Read the model definition and answer for the solid it produces. Units are mm, in the model's axes. A direction names the side the tool comes from. Give positions to 0.01 mm unless a question says otherwise; leave off trailing zeros. Write each loop counter-clockwise with the first axis right and the second up, starting at its lowest first coordinate (ties: lowest second). Pieces come first, ordered by that corner, then holes. Notation, with made-up numbers: (40, 23.5) -> (67, 23.5) arc R17 cw to (67, 37.5) -> close; hole circle Ø2 at (-40, 40.5). An arc over 180 degrees is marked (long way). Answer as CSV lines item,"result". Start each with the question number.
1. Given pin 1 (1.5 mm diameter, centred on x = 151.5, y = 38.5, fed in from -Z), flat-ended and moving along its own axis, determine where the tip first touches the part or whether it passes through.
2. The part is cut by section B-B, the plane y = 27.5. Determine the outline of the cut face in (x, z).
3. A tool of negligible diameter and unlimited length cuts with its end or side. For faces 4 (the flat face through (76, 77, 4)), 5 (the flat face through (92, 72, 3)), 6 (the cylindrical face through (40.455, 74.535, 4.354)), from which of +Z, -Z, +X, -X, +Y, -Y can it reach the whole face along a straight path? Write none if from no direction.
4. The part is cut by section A-A, the plane x = 121.5. Determine the outline of the cut face in (y, z), and give its area (3 significant figures).
5. For a pull along Y with two mould halves and no side action, classify faces 1 (the flat face through (0, 38, 4)), 2 (the flat face through (78.25, 39, 3)), 3 (the flat face through (76, 0, 4)) as pulls with the +Y half, pulls with the -Y half, needs draft (parallel to the pull), parting line crosses it, or undercut.
6. Find the intervals of material crossed by line 1 (X direction, y = 51, z = 4.5); line 2 (Y direction, x = 126.25, z = 3.2); line 3 (Y direction, x = 151.5, z = 3.85), in increasing order.
from build123d import *

# Parameters (mm, degrees)
F0_W      = 154
F0_H      = 77
F1_DEPTH  = 8.127
F3_R      = 1.25
F4_DEPTH  = 5
F5_R      = 1.25
F6_DEPTH  = 5
F7_R      = 1.25
F8_DEPTH  = 5
F9_R      = 1.25
F10_DEPTH = 5
F11_R     = 1.25
F12_DEPTH = 5
F13_R     = 1.25
F14_DEPTH = 5
F15_R     = 1.25
F16_DEPTH = 5
F17_R     = 1.25
F18_DEPTH = 5
F19_R     = 1.25
F20_DEPTH = 5
F21_R     = 1.25
F22_DEPTH = 5
F23_R     = 1.25
F24_DEPTH = 5
F25_R     = 1.25
F26_DEPTH = 5
F27_R     = 1.25
F28_DEPTH = 5
F29_R     = 1.25
F30_DEPTH = 5
F31_R     = 1.25
F32_DEPTH = 5
F33_R     = 1.25
F34_DEPTH = 5
F35_R     = 1.25
F36_DEPTH = 5
F37_R     = 1.25
F38_DEPTH = 5
F39_R     = 1.25
F40_DEPTH = 5
F41_R     = 1.25
F42_DEPTH = 5
F2_W      = 140
F2_H      = 67
F43_DEPTH = 5.127
F45_W     = 2
F45_H     = 67
F46_DEPTH = 0.254
F47_W     = 2
F47_H     = 67
F48_DEPTH = 0.254
F49_R     = 2.05
F50_DEPTH = 5
F51_R     = 2.05
F52_DEPTH = 5
F53_W     = 4.1
F53_H     = 2.304
F54_DEPTH = 5
F55_W     = 4.1
F55_H     = 2.304
F56_DEPTH = 5
F57_R     = 1.25
F58_DEPTH = 2.5
F44_W     = 2.5
F44_H     = 67
F59_DEPTH = 4.873
F60_W     = 2.5
F60_H     = 6.7
F61_DEPTH = 0.723


with BuildPart() as f1:
    # F0 (on Top) → F1 (new body)
    with BuildSketch(Plane.XY):
        with Locations((77, 38.5)):
            Rectangle(F0_W, F0_H)
    extrude(amount=F1_DEPTH)

    # F3 (on face) → F4 (cut)
    with BuildSketch(Plane(origin=(0, 0, 0), x_dir=(1, 0, 0), z_dir=(0, 0, -1))):
        with Locations((2.5, -2.5)):
            Circle(F3_R)
    extrude(amount=-F4_DEPTH, mode=Mode.SUBTRACT)

    # F5 (on face) → F6 (cut)
    with BuildSketch(Plane(origin=(0, 0, 0), x_dir=(1, 0, 0), z_dir=(0, 0, -1))):
        with Locations((2.5, -22)):
            Circle(F5_R)
    extrude(amount=-F6_DEPTH, mode=Mode.SUBTRACT)

    # F7 (on face) → F8 (cut)
    with BuildSketch(Plane(origin=(0, 0, 0), x_dir=(1, 0, 0), z_dir=(0, 0, -1))):
        with Locations((151.5, -2.5)):
            Circle(F7_R)
    extrude(amount=-F8_DEPTH, mode=Mode.SUBTRACT)

    # F9 (on face) → F10 (cut)
    with BuildSketch(Plane(origin=(0, 0, 0), x_dir=(1, 0, 0), z_dir=(0, 0, -1))):
        with Locations((151.5, -22)):
            Circle(F9_R)
    extrude(amount=-F10_DEPTH, mode=Mode.SUBTRACT)

    # F11 (on face) → F12 (cut)
    with BuildSketch(Plane(origin=(0, 0, 0), x_dir=(1, 0, 0), z_dir=(0, 0, -1))):
        with Locations((2.5, -38.5)):
            Circle(F11_R)
    extrude(amount=-F12_DEPTH, mode=Mode.SUBTRACT)

    # F13 (on face) → F14 (cut)
    with BuildSketch(Plane(origin=(0, 0, 0), x_dir=(1, 0, 0), z_dir=(0, 0, -1))):
        with Locations((151.5, -38.5)):
            Circle(F13_R)
    extrude(amount=-F14_DEPTH, mode=Mode.SUBTRACT)

    # F15 (on face) → F16 (cut)
    with BuildSketch(Plane(origin=(0, 0, 0), x_dir=(1, 0, 0), z_dir=(0, 0, -1))):
        with Locations((2.5, -55)):
            Circle(F15_R)
    extrude(amount=-F16_DEPTH, mode=Mode.SUBTRACT)

    # F17 (on face) → F18 (cut)
    with BuildSketch(Plane(origin=(0, 0, 0), x_dir=(1, 0, 0), z_dir=(0, 0, -1))):
        with Locations((151.5, -55)):
            Circle(F17_R)
    extrude(amount=-F18_DEPTH, mode=Mode.SUBTRACT)

    # F19 (on face) → F20 (cut)
    with BuildSketch(Plane(origin=(0, 0, 0), x_dir=(1, 0, 0), z_dir=(0, 0, -1))):
        with Locations((2.5, -74.5)):
            Circle(F19_R)
    extrude(amount=-F20_DEPTH, mode=Mode.SUBTRACT)

    # F21 (on face) → F22 (cut)
    with BuildSketch(Plane(origin=(0, 0, 0), x_dir=(1, 0, 0), z_dir=(0, 0, -1))):
        with Locations((151.5, -74.5)):
            Circle(F21_R)
    extrude(amount=-F22_DEPTH, mode=Mode.SUBTRACT)

    # F23 (on face) → F24 (cut)
    with BuildSketch(Plane(origin=(0, 0, 0), x_dir=(1, 0, 0), z_dir=(0, 0, -1))):
        with Locations((26.25, -2.5)):
            Circle(F23_R)
    extrude(amount=-F24_DEPTH, mode=Mode.SUBTRACT)

    # F25 (on face) → F26 (cut)
    with BuildSketch(Plane(origin=(0, 0, 0), x_dir=(1, 0, 0), z_dir=(0, 0, -1))):
        with Locations((26.25, -74.5)):
            Circle(F25_R)
    extrude(amount=-F26_DEPTH, mode=Mode.SUBTRACT)

    # F27 (on face) → F28 (cut)
    with BuildSketch(Plane(origin=(0, 0, 0), x_dir=(1, 0, 0), z_dir=(0, 0, -1))):
        with Locations((51.25, -2.5)):
            Circle(F27_R)
    extrude(amount=-F28_DEPTH, mode=Mode.SUBTRACT)

    # F29 (on face) → F30 (cut)
    with BuildSketch(Plane(origin=(0, 0, 0), x_dir=(1, 0, 0), z_dir=(0, 0, -1))):
        with Locations((76.25, -2.5)):
            Circle(F29_R)
    extrude(amount=-F30_DEPTH, mode=Mode.SUBTRACT)

    # F31 (on face) → F32 (cut)
    with BuildSketch(Plane(origin=(0, 0, 0), x_dir=(1, 0, 0), z_dir=(0, 0, -1))):
        with Locations((51.25, -74.5)):
            Circle(F31_R)
    extrude(amount=-F32_DEPTH, mode=Mode.SUBTRACT)

    # F33 (on face) → F34 (cut)
    with BuildSketch(Plane(origin=(0, 0, 0), x_dir=(1, 0, 0), z_dir=(0, 0, -1))):
        with Locations((101.25, -2.5)):
            Circle(F33_R)
    extrude(amount=-F34_DEPTH, mode=Mode.SUBTRACT)

    # F35 (on face) → F36 (cut)
    with BuildSketch(Plane(origin=(0, 0, 0), x_dir=(1, 0, 0), z_dir=(0, 0, -1))):
        with Locations((76.25, -74.5)):
            Circle(F35_R)
    extrude(amount=-F36_DEPTH, mode=Mode.SUBTRACT)

    # F37 (on face) → F38 (cut)
    with BuildSketch(Plane(origin=(0, 0, 0), x_dir=(1, 0, 0), z_dir=(0, 0, -1))):
        with Locations((126.25, -2.5)):
            Circle(F37_R)
    extrude(amount=-F38_DEPTH, mode=Mode.SUBTRACT)

    # F39 (on face) → F40 (cut)
    with BuildSketch(Plane(origin=(0, 0, 0), x_dir=(1, 0, 0), z_dir=(0, 0, -1))):
        with Locations((101.25, -74.5)):
            Circle(F39_R)
    extrude(amount=-F40_DEPTH, mode=Mode.SUBTRACT)

    # F41 (on face) → F42 (cut)
    with BuildSketch(Plane(origin=(0, 0, 0), x_dir=(1, 0, 0), z_dir=(0, 0, -1))):
        with Locations((126.25, -74.5)):
            Circle(F41_R)
    extrude(amount=-F42_DEPTH, mode=Mode.SUBTRACT)

    # F2 (on Top) → F43 (cut)
    with BuildSketch(Plane.XY):
        with Locations((77, 38.5)):
            Rectangle(F2_W, F2_H)
    extrude(amount=F43_DEPTH, mode=Mode.SUBTRACT)

    # F45 (on face) → F46 (cut)
    with BuildSketch(Plane(origin=(0, 0, 0), x_dir=(1, 0, 0), z_dir=(0, 0, -1))):
        with Locations((6, -38.5)):
            Rectangle(F45_W, F45_H)
    extrude(amount=-F46_DEPTH, mode=Mode.SUBTRACT)

    # F47 (on face) → F48 (cut)
    with BuildSketch(Plane(origin=(0, 0, 0), x_dir=(1, 0, 0), z_dir=(0, 0, -1))):
        with Locations((148, -38.5)):
            Rectangle(F47_W, F47_H)
    extrude(amount=-F48_DEPTH, mode=Mode.SUBTRACT)

    # F49 (on face) → F50 (cut)
    with BuildSketch(Plane(origin=(0, 77, 0), x_dir=(-1, 0, 0), z_dir=(0, 1, 0))):
        with Locations((-40.5, 2.304)):
            Circle(F49_R)
    extrude(amount=-F50_DEPTH, mode=Mode.SUBTRACT)

    # F51 (on face) → F52 (cut)
    with BuildSketch(Plane(origin=(0, 77, 0), x_dir=(-1, 0, 0), z_dir=(0, 1, 0))):
        with Locations((-113.5, 2.304)):
            Circle(F51_R)
    extrude(amount=-F52_DEPTH, mode=Mode.SUBTRACT)

    # F53 (on face) → F54 (cut)
    with BuildSketch(Plane(origin=(0, 77, 0), x_dir=(-1, 0, 0), z_dir=(0, 1, 0))):
        with Locations((-113.5, 1.152)):
            Rectangle(F53_W, F53_H)
    extrude(amount=-F54_DEPTH, mode=Mode.SUBTRACT)

    # F55 (on face) → F56 (cut)
    with BuildSketch(Plane(origin=(0, 77, 0), x_dir=(-1, 0, 0), z_dir=(0, 1, 0))):
        with Locations((-40.5, 1.152)):
            Rectangle(F55_W, F55_H)
    extrude(amount=-F56_DEPTH, mode=Mode.SUBTRACT)

    # F57 (on face) → F58 (cut)
    with BuildSketch(Plane(origin=(0, 77, 0), x_dir=(-1, 0, 0), z_dir=(0, 1, 0))):
        with Locations((-36.2, 6.604)):
            Circle(F57_R)
        with Locations((-44.8, 6.604)):
            Circle(F57_R)
        with Locations((-117.8, 6.604)):
            Circle(F57_R)
        with Locations((-109.2, 6.604)):
            Circle(F57_R)
    extrude(amount=-F58_DEPTH, mode=Mode.SUBTRACT)

    # F44 (on face) → F59 (join)
    with BuildSketch(Plane(origin=(0, 0, 5.127), x_dir=(1, 0, 0), z_dir=(0, 0, -1))):
        with Locations((77, -38.5)):
            Rectangle(F44_W, F44_H)
    extrude(amount=F59_DEPTH)

    # F60 (on face) → F61 (cut)
    with BuildSketch(Plane(origin=(0, 0, 0.254), x_dir=(1, 0, 0), z_dir=(0, 0, -1))):
        with Locations((77, -38.5)):
            Rectangle(F60_W, F60_H)
    extrude(amount=-F61_DEPTH, mode=Mode.SUBTRACT)


solid = f1.part
Results found:
1,pin 1,"stops at z = 5"
2,outline,"(0, 0) -> (5, 0) -> (5, 0.25) -> (7, 0.25) -> (7, 5.13) -> (75.75, 5.13) -> (75.75, 0.25) -> (78.25, 0.25) -> (78.25, 5.13) -> (147, 5.13) -> (147, 0.25) -> (149, 0.25) -> (149, 0) -> (154, 0) -> (154, 8.13) -> (0, 8.13) -> close"
3,face 4,"+Z, -Z, +X, -X, +Y"
3,face 5,"-Z"
3,face 6,"-Z, +Y"
4,outline,"(0, 0) -> (5, 0) -> (5, 5.13) -> (72, 5.13) -> (72, 0) -> (77, 0) -> (77, 8.13) -> (0, 8.13) -> close"
4,area,"282 mm²"
5,face 1,"needs draft"
5,face 2,"undercut"
5,face 3,"pulls with the -Y half"
6,line 1,"x = 0 to 7, 75.75 to 78.25, 147 to 154"
6,line 2,"y = 0 to 1.25, 3.75 to 5, 72 to 73.25, 75.75 to 77"
6,line 3,"y = 0 to 1.25, 3.75 to 20.75, 23.25 to 37.25, 39.75 to 53.75, 56.25 to 73.25, 75.75 to 77"
